Design review of the part built by this model. Coordinates are the model's own, in mm. Face numbers are marked on the shaded views. A direction names the side the tool comes from. Give positions to 0.01 mm unless a question says otherwise; leave off trailing zeros. Write each loop counter-clockwise with the first axis right and the second up, starting at its lowest first coordinate (ties: lowest second). Pieces come first, ordered by that corner, then holes. Notation, with made-up numbers: (51.25, -3) -> (79.25, -3) arc R21 ccw to (79.25, 17) -> close; hole circle Ø1 at (71, 5.5). An arc over 180 degrees is marked (long way). Return JSON: item names as keys, results as strings. Group by question number.
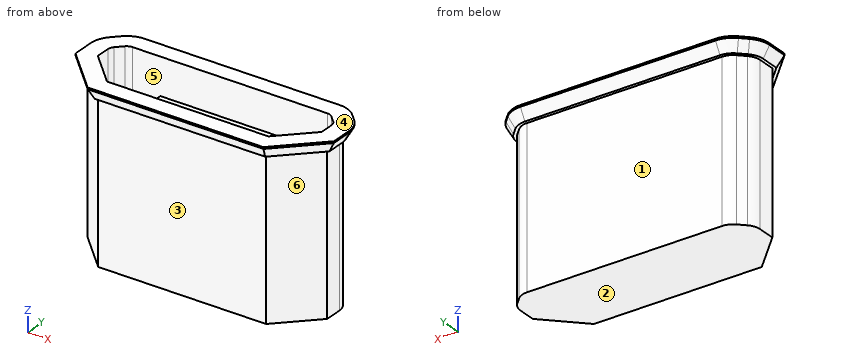
Autodesk Inventor part; units mm, degrees
ref_plane "Work Plane1" through (9.2852, 10.0149, 0) normal (-1, 0, 0) x (0, 0, 1)
ref_plane "YZ Plane" through (0, 0, 0) normal (1, 0, 0) x (0, 1, 0)
ref_plane "XZ Plane" through (0, 0, 0) normal (0, 1, 0) x (-1, 0, 0)
sketch "Sketch1" plane through (0, 0, 0) normal (0, 0, 1) x (1, 0, 0)
  line L0 (6.1823, 11.2749) -> (12.3881, 11.2749)
  line L1 (13.0952, 10.5678) -> (13.0952, 10.0149)
  line L2 (11.9552, 8.8749) -> (6.6152, 8.8749)
  line L3 (5.4752, 10.0149) -> (5.4752, 10.5678)
  line L4 (5.4752, 10.0149) -> (6.6152, 8.8749)
  line L5 (11.9552, 8.8749) -> (13.0952, 10.0149)
  line L6 (5.6217, 10.9213) -> (5.8288, 11.1284)
  line L7 (12.7417, 11.1284) -> (12.9488, 10.9213)
  arc A0 (6.1823, 11.2749) -> (5.8288, 11.1284) centre (6.1823, 10.7749) ccw
  arc A1 (5.6217, 10.9213) -> (5.4752, 10.5678) centre (5.9752, 10.5678) ccw
  arc A2 (12.7417, 11.1284) -> (12.3881, 11.2749) centre (12.3881, 10.7749) ccw
  arc A3 (13.0952, 10.5678) -> (12.9488, 10.9213) centre (12.5952, 10.5678) ccw
  line L8 (12.3881, 11.0249) -> (6.1823, 11.0249)
  arc A4 (6.1823, 11.0249) -> (6.0055, 10.9517) centre (6.1823, 10.7749) ccw
  line L9 (6.0055, 10.9517) -> (5.7984, 10.7446)
  arc A5 (5.7984, 10.7446) -> (5.7252, 10.5678) centre (5.9752, 10.5678) ccw
  line L10 (5.7252, 10.5678) -> (5.7252, 10.1184)
  line L11 (5.7252, 10.1184) -> (6.7188, 9.1249)
  line L12 (6.7188, 9.1249) -> (11.8517, 9.1249)
  line L13 (11.8517, 9.1249) -> (12.8452, 10.1184)
  line L14 (12.8452, 10.1184) -> (12.8452, 10.5678)
  arc A6 (12.8452, 10.5678) -> (12.772, 10.7446) centre (12.5952, 10.5678) ccw
  line L15 (12.772, 10.7446) -> (12.5649, 10.9517)
  arc A7 (12.5649, 10.9517) -> (12.3881, 11.0249) centre (12.3881, 10.7749) ccw
  point P0 (0, 0)
  point P1 (13.0952, 8.8749)
  point P2 (5.4752, 8.8749)
  point P3 (5.4752, 11.2749)
  point P4 (13.0952, 11.2749)
  point P5 (5.4752, 10.7749)
  point P6 (5.9752, 11.2749)
  point P7 (12.5952, 11.2749)
  point P8 (13.0952, 10.7749)
  dimension "d0" = 7.62
  dimension "d1" = 2.4
  dimension "d3" = 1.14
  dimension "d4" = 1.14
  dimension "d5" = 1.14
  dimension "d6" = 1.14
  dimension "d7" = 0.5
  dimension "d8" = 0.5
  dimension "d9" = 0.5
  dimension "d10" = 0.5
  dimension "d11" = 0.5
  dimension "d12" = 0.25
extrude "Extrusion1" add sketch "Sketch1" against normal blind 5.42
sketch "Sketch2" plane through (0, 0, -5.42) normal (0, 0, -1) x (-1, 0, 0)
  line L0 (-12.8452, 10.1184) -> (-12.8452, 10.5678)
  arc A0 (-12.772, 10.7446) -> (-12.8452, 10.5678) centre (-12.5952, 10.5678) ccw
  line L1 (-12.772, 10.7446) -> (-12.5649, 10.9517)
  arc A1 (-12.3881, 11.0249) -> (-12.5649, 10.9517) centre (-12.3881, 10.7749) ccw
  line L2 (-12.3881, 11.0249) -> (-6.1823, 11.0249)
  line L3 (-11.8517, 9.1249) -> (-12.8452, 10.1184)
  line L4 (-6.7188, 9.1249) -> (-11.8517, 9.1249)
  line L5 (-5.7252, 10.1184) -> (-6.7188, 9.1249)
  line L6 (-5.7252, 10.5678) -> (-5.7252, 10.1184)
  arc A2 (-5.7252, 10.5678) -> (-5.7984, 10.7446) centre (-5.9752, 10.5678) ccw
  arc A3 (-6.0055, 10.9517) -> (-6.1823, 11.0249) centre (-6.1823, 10.7749) ccw
  line L7 (-6.0055, 10.9517) -> (-5.7984, 10.7446)
extrude "Extrusion2" add sketch "Sketch2" against normal blind 0.2
sketch "Sketch3" plane through (0, 0, -5.22) normal (0, 0, 1) x (1, 0, 0)
  line L0 (7.2852, 10.7249) -> (11.2852, 10.7249)
  line L1 (11.2852, 10.7249) -> (11.2852, 10.0149)
  line L2 (11.2852, 10.0149) -> (7.2852, 10.0149)
  line L3 (7.2852, 10.0149) -> (7.2852, 10.7249)
  line L4 (6.1823, 11.0249) -> (12.3881, 11.0249)
  line L5 (9.2852, 11.0249) -> (9.2852, 10.7249)
  point P0 (9.2852, 10.3699)
  point P1 (9.2852, 10.7249)
  dimension "d17" = 4
  dimension "d18" = 0.71
  dimension "d19" = 0.3
extrude "Extrusion3" add sketch "Sketch3" along normal blind 4.25
ref_plane "Work Plane1" through (9.2852, 10.0149, 0) normal (-1, 0, 0) x (0, 0, 1)
sketch "Sketch4" plane through (0, 0, 0) normal (0, 0, 1) x (1, 0, 0)
  arc A0 (5.6217, 10.9213) -> (5.4752, 10.5678) centre (5.9752, 10.5678) ccw
  line L0 (5.4752, 10.5678) -> (5.4752, 10.0149)
  line L1 (5.4752, 10.0149) -> (6.6152, 8.8749)
  line L2 (6.6152, 8.8749) -> (11.9552, 8.8749)
  line L3 (11.9552, 8.8749) -> (13.0952, 10.0149)
  line L4 (13.0952, 10.0149) -> (13.0952, 10.5678)
  arc A1 (13.0952, 10.5678) -> (12.9488, 10.9213) centre (12.5952, 10.5678) ccw
  line L5 (12.9488, 10.9213) -> (12.7417, 11.1284)
  arc A2 (12.7417, 11.1284) -> (12.3881, 11.2749) centre (12.3881, 10.7749) ccw
  line L6 (12.3881, 11.2749) -> (6.1823, 11.2749)
  arc A3 (6.1823, 11.2749) -> (5.8288, 11.1284) centre (6.1823, 10.7749) ccw
  line L7 (5.8288, 11.1284) -> (5.6217, 10.9213)
  line L8 (6.1823, 11.5749) -> (12.3881, 11.5749)
  arc A4 (12.9538, 11.3406) -> (12.3881, 11.5749) centre (12.3881, 10.7749) ccw
  line L9 (12.9538, 11.3406) -> (13.1609, 11.1335)
  arc A5 (13.3952, 10.5678) -> (13.1609, 11.1335) centre (12.5952, 10.5678) ccw
  line L10 (13.3952, 10.5678) -> (13.3952, 9.8906)
  line L11 (13.3952, 9.8906) -> (12.0795, 8.5749)
  line L12 (12.0795, 8.5749) -> (6.491, 8.5749)
  line L13 (6.491, 8.5749) -> (5.1752, 9.8906)
  line L14 (5.1752, 9.8906) -> (5.1752, 10.5678)
  arc A6 (5.4095, 11.1335) -> (5.1752, 10.5678) centre (5.9752, 10.5678) ccw
  line L15 (5.4095, 11.1335) -> (5.6166, 11.3406)
  arc A7 (6.1823, 11.5749) -> (5.6166, 11.3406) centre (6.1823, 10.7749) ccw
  dimension "d22" = 0.3
extrude "Extrusion4" add sketch "Sketch4" against normal blind 0.4
chamfer "Chamfer1" distance 0.2 angle 60 12 edges at (12.6943, 11.514, -0.4) (13.0573, 11.237, -0.4) (13.3343, 10.8739, -0.4) (13.3952, 10.2292, -0.4) (9.2852, 11.5749, -0.4) (5.8762, 11.514, -0.4) (5.5131, 11.237, -0.4) (5.2361, 10.8739, -0.4) (5.1752, 10.2292, -0.4) (12.7373, 9.2328, -0.4) (5.8331, 9.2328, -0.4) (9.2852, 8.5749, -0.4) measured on face at (10.3195, 11.4749, -0.4)
properties part number "USB Port"
Q1. Tool access review of the marked faces 1, 2 and 3: name each direction out of +Z, -Z, +X, -X, +Y, -Y from which nothing blocks a thin tool from reaching the whole face with its end or side.
Q2. Insertion check: pin 1 (0.5 mm diameter, centred on y = 10.5, z = -3, fed in from +X); pin 2 (1.5 mm diameter, centred on x = 8, y = 10, fed in from +Z). Each pin has a flat end and moves straight along its axis. Give the tip position at first contact, or say it passes through.
Q3. Take a section at B-B, the plane x = 7. Give the boundary of the cut face in (y, z), plus the area to 3 significant figures.
Q4. Mouldability with a two-part tool opening along Y and no side actions: class the marked faces 4, 5 and 6 as +Y half, -Y half, draft (parallel to the pull), parting line (faces both ways), or undercut.
Q5. Take a section at D-D, the plane x = 10.5. Give the boundary of the cut face in (y, z), plus the area to 3 significant figures.
Q6. Take a section at A-A, the plane z = -2.1. Give the boundary of the cut face in (x, y), plus the area to 3 significant figures.
Q7. For L1, parallel to X at y = 10.35, z = -2.8; L2, parallel to Y at x = 10.25, z = -1.9; L3, parallel to Y at x = 11.5, z = -0.6, list the stretches that pass through material, from the lowest coordinate up. Write a range as from..to.
Q8. Take a section at C-C, the plane z = -0.8. Give the boundary of the cut face in (x, y), plus the area to 3 significant figures.
Final values:
{
 "1": {"face 1": "-Z, +X, -X, +Y", "face 2": "-Z, +X, -X, +Y, -Y", "face 3": "-Z, +X, -X, -Y"},
 "2": {"pin 1": "stops at x = 13.1", "pin 2": "stops at z = -0.97"},
 "3": {"outline": "(8.57, -0.05) -> (8.77, -0.4) -> (8.87, -0.4) -> (8.87, -5.42) -> (11.27, -5.42) -> (11.27, -0.4) -> (11.37, -0.4) -> (11.57, -0.05) -> (11.57, 0) -> (11.02, 0) -> (11.02, -5.22) -> (9.12, -5.22) -> (9.12, 0) -> (8.57, 0) -> close", "area": "3.26 mm²"},
 "4": {"face 4": "draft", "face 5": "undercut", "face 6": "-Y half"},
 "5": {"outline": "(8.57, -0.05) -> (8.77, -0.4) -> (8.87, -0.4) -> (8.87, -5.42) -> (11.27, -5.42) -> (11.27, -0.4) -> (11.37, -0.4) -> (11.57, -0.05) -> (11.57, 0) -> (11.02, 0) -> (11.02, -5.22) -> (10.72, -5.22) -> (10.72, -0.97) -> (10.01, -0.97) -> (10.01, -5.22) -> (9.12, -5.22) -> (9.12, 0) -> (8.57, 0) -> close", "area": "6.28 mm²"},
 "6": {"outline": "(5.48, 10.01) -> (6.62, 8.87) -> (11.96, 8.87) -> (13.1, 10.01) -> (13.1, 10.57) arc R0.5 ccw to (12.95, 10.92) -> (12.74, 11.13) arc R0.5 ccw to (12.39, 11.27) -> (6.18, 11.27) arc R0.5 ccw to (5.83, 11.13) -> (5.62, 10.92) arc R0.5 ccw to (5.48, 10.57) -> close; (7.29, 10.01) -> (11.29, 10.01) -> (11.29, 10.72) -> (7.29, 10.72) -> close; hole (5.73, 10.12) -> (6.72, 9.12) -> (11.85, 9.12) -> (12.85, 10.12) -> (12.85, 10.57) arc R0.25 ccw to (12.77, 10.74) -> (12.56, 10.95) arc R0.25 ccw to (12.39, 11.02) -> (6.18, 11.02) arc R0.25 ccw to (6.01, 10.95) -> (5.8, 10.74) arc R0.25 ccw to (5.73, 10.57) -> close", "area": "7.15 mm²"},
 "7": {"L1": "x = 5.48..5.73, 7.29..11.29, 12.85..13.1", "L2": "y = 8.87..9.12, 10.01..10.72, 11.02..11.27", "L3": "y = 8.87..9.12, 11.02..11.27"},
 "8": {"outline": "(5.48, 10.01) -> (6.62, 8.87) -> (11.96, 8.87) -> (13.1, 10.01) -> (13.1, 10.57) arc R0.5 ccw to (12.95, 10.92) -> (12.74, 11.13) arc R0.5 ccw to (12.39, 11.27) -> (6.18, 11.27) arc R0.5 ccw to (5.83, 11.13) -> (5.62, 10.92) arc R0.5 ccw to (5.48, 10.57) -> close; hole (5.73, 10.12) -> (6.72, 9.12) -> (11.85, 9.12) -> (12.85, 10.12) -> (12.85, 10.57) arc R0.25 ccw to (12.77, 10.74) -> (12.56, 10.95) arc R0.25 ccw to (12.39, 11.02) -> (6.18, 11.02) arc R0.25 ccw to (6.01, 10.95) -> (5.8, 10.74) arc R0.25 ccw to (5.73, 10.57) -> close", "area": "4.31 mm²"}
}
